For this review, take the finished solid that the model builds, in its own axes (mm). Face numbers are marked on the shaded views. Round coordinates to 2 decimals unless told otherwise and drop trailing zeros. Loops run counter-clockwise (first coordinate to the right, second up) from the corner with the lowest first, then second, coordinate; pieces in that order, holes last.
1) Wall thickness on L1, parallel to X at y = -1.75, z = 0; L2, parallel to X at y = 10, z = -6; L3, parallel to Z at x = -12, y = 3: over which ranges is each line inside the solid? List them lowest first.
2) Mouldability with a two-part tool opening along Z and no side actions: class the marked faces 1, 2 and 3 as pulls with the +Z half, pulls with the -Z half, needs draft (parallel to the pull), parting line crosses it, or undercut.
3) Insertion check: pin 1 (2 mm diameter, centred on y = -6.5, z = 11, fed in from -X); pin 2 (2 mm diameter, centred on y = 7.5, z = -19, fed in from -X); pin 3 (5 mm diameter, centred on y = -7, z = -7.5, fed in from +X). Each pin has a flat end and moves straight along its axis. Give the tip position at first contact, or say it passes through.
4) Take a section at A-A (y = 5). State the section outline as (x, z) points, then the cut area to 3 significant figures.
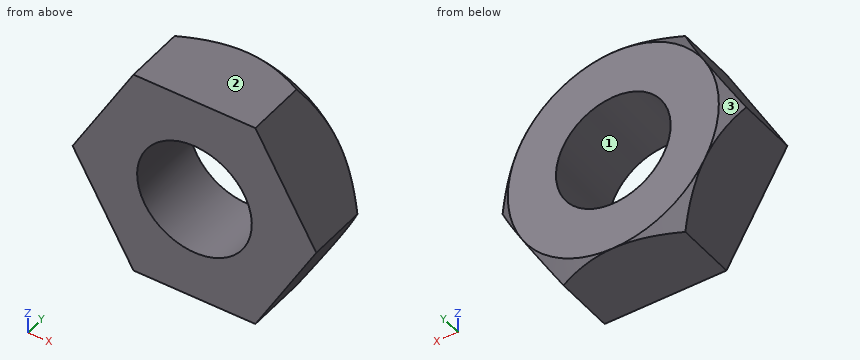
```python
from build123d import *

# Parameters (mm, degrees)
SKETCH1_R           = 18.75
BOSS_EXTRUDE1_DEPTH = 12.5
SKETCH2_OUTSIDE_W   = 221.996
SKETCH2_OUTSIDE_H   = 211.322
SKETCH2_OUTSIDE_R   = 34.5
CUT_EXTRUDE1_DEPTH  = 59.328809348
CUT_EXTRUDE1_DRAFT  = -45


with BuildPart() as part:
    # Sketch1 → Boss-Extrude1 (new, symmetric)
    with BuildSketch(Plane(origin=(0, 0, 0), x_dir=(1, 0, 0), z_dir=(0, 1, 0))):
        Polygon((39.837168574, 0), (19.918584287, 34.5), (-19.918584287, 34.5), (-39.837168574, 0), (-19.918584287, -34.5), (19.918584287, -34.5), align=None)
        with Locations(Location((0, 0, 0), (0, 0, 270))):
            Circle(SKETCH1_R, mode=Mode.SUBTRACT)
    extrude(amount=BOSS_EXTRUDE1_DEPTH, both=True)


with BuildPart() as cut_extrude1_tool:
    # Sketch2 outside → Cut-Extrude1 (with draft: the straight prism first)
    with BuildSketch(Plane(origin=(0, 12.5, 0), x_dir=(1, 0, 0), z_dir=(0, 1, 0))):
        Rectangle(SKETCH2_OUTSIDE_W, SKETCH2_OUTSIDE_H)
        Circle(SKETCH2_OUTSIDE_R, mode=Mode.SUBTRACT)
    extrude(amount=-CUT_EXTRUDE1_DEPTH)
    # Cut-Extrude1: the draft: its side faces are tilted about the plane it starts from
    cut_extrude1_sides = [cut_extrude1_tool.faces().sort_by_distance(p)[0] for p in [
        (0, -17.164404674, 105.661),
        (110.998, -17.164404674, 0),
        (0, -17.164404674, -105.661),
        (-110.998, -17.164404674, 0),
        (-34.5, -17.164404674, 0),
    ]]
    draft(cut_extrude1_sides, Plane(origin=(0, 12.5, 0), x_dir=(1, 0, 0), z_dir=(0, 1, 0)), CUT_EXTRUDE1_DRAFT)


with BuildPart() as part_1:
    add(part.part)

    # Cut-Extrude1: cut by cut_extrude1_tool
    add(cut_extrude1_tool.part, mode=Mode.SUBTRACT)


solid = part_1.part
```
Response:
1. L1: x = -39.84 to -18.75, 18.75 to 39.84
1. L2: x = -36.37 to -17.76, 17.76 to 36.37
1. L3: z = -34.5 to -14.41, 14.41 to 34.5
2. face 1: undercut
2. face 2: pulls with the +Z half
2. face 3: parting line crosses it
3. pin 1: stops at x = -34.06
3. pin 2: stops at x = -29.44
3. pin 3: stops at x = 36.95
4. outline: (-39.84, 0) - (-19.92, -34.5) - (19.92, -34.5) - (39.84, 0) - (19.92, 34.5) - (-19.92, 34.5) - close; hole circle Ø37.5 at (0, 0)
4. area: 3,020 mm2
